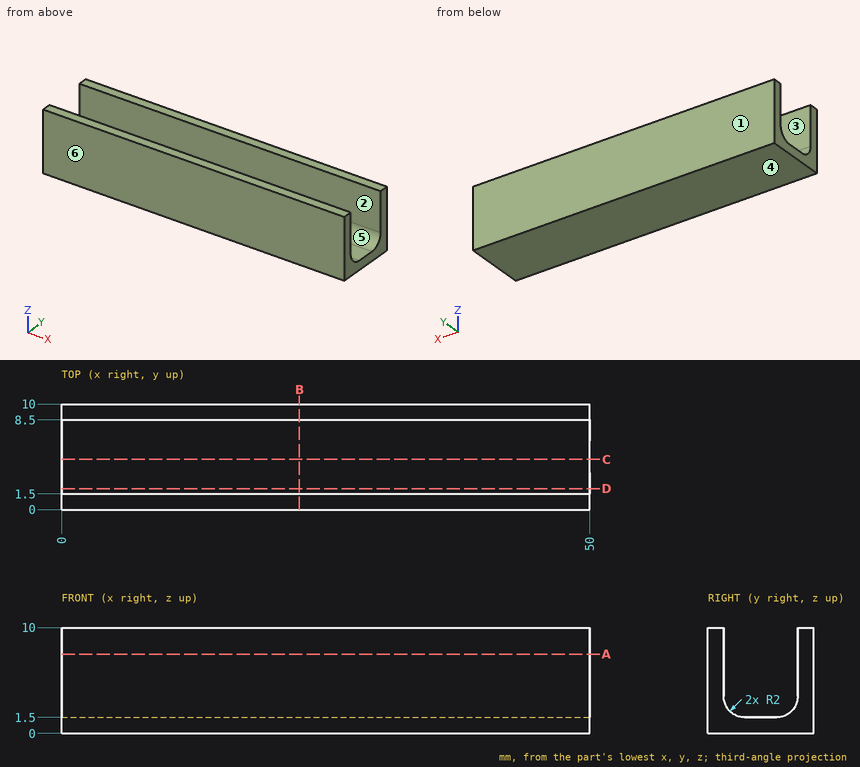
Input: dimensioned drawing with shaded views. Units: mm. Origin: part minimum x, y, z. A direction names the side the tool comes from. Round coordinates to 2 decimals unless told otherwise and drop trailing zeros. Loops run counter-clockwise (first coordinate to the right, second up) from the corner with the lowest first, then second, coordinate; pieces in that order, holes last. Notation, with made-up numbers: (42.25, -13.75) -> (51.25, -13.75) arc R16 ccw to (51.25, 2.25) -> close; hole circle Ø2 at (40, 13.5). An arc over 180 degrees is marked (long way). Answer as a JSON object with one key per item and string values. Group by question number.
Q1. Access query for the marked faces 1 and 2. Directions: +Z, -Z, +X, -X, +Y, -Y. A direction counts if a zero-diameter tool reaches every point of the face in a straight line with its end or side. Return the directions, or none.
Q2. Ray query, line 1 (Y direction, x = 21, z = 6.25); line 2 (Z direction, x = 47, y = 3.75); line 3 (Y direction, x = 17.5, z = 2.5). Return the intervals inside material, ascending. Write a range as from..to.
Q3. Section query A-A (z = 7.5). Output: boundary loops of the cut face in (x, y).
Q4. Section query B-B (x = 22.5). Output: boundary loops of the cut face in (y, z), plus the area to 3 significant figures.
Q5. Mould query, pull axis Y, two halves, no side actions, for the marked faces 3, 4, 5 and 6. Classes: pulls with the +Y half, pulls with the -Y half, needs draft (parallel to the pull), parting line crosses it, or undercut.
Q6. Contact query for a flat-ended pin moving along its axis: P1, Ø2.5, axis at x = 15, y = 5, coming from the +Z side. Output: stop coordinate, or through.
Q7. Section query D-D (y = 2). Output: boundary loops of the cut face in (x, z).
Q8. Section query C-C (y = 4.75). Output: boundary loops of the cut face in (x, z), plus the area to 3 significant figures.
Completed:
{
 "1": {"face 1": "+Z, -Z, +X, -X, +Y", "face 2": "+Z, +X, -X"},
 "2": {"line 1": "0..1.5, 8.5..10", "line 2": "0..1.5", "line 3": "0..1.77, 8.23..10"},
 "3": {"outline": "(0, 0) -> (50, 0) -> (50, 1.5) -> (0, 1.5) -> close; (0, 8.5) -> (50, 8.5) -> (50, 10) -> (0, 10) -> close"},
 "4": {"outline": "(0, 0) -> (10, 0) -> (10, 10) -> (8.5, 10) -> (8.5, 3.5) arc R2 cw to (6.5, 1.5) -> (3.5, 1.5) arc R2 cw to (1.5, 3.5) -> (1.5, 10) -> (0, 10) -> close", "area": "42.2 mm²"},
 "5": {"face 3": "undercut", "face 4": "needs draft", "face 5": "undercut", "face 6": "pulls with the -Y half"},
 "6": {"P1": "z = 1.5"},
 "7": {"outline": "(0, 0) -> (50, 0) -> (50, 2.18) -> (0, 2.18) -> close"},
 "8": {"outline": "(0, 0) -> (50, 0) -> (50, 1.5) -> (0, 1.5) -> close", "area": "75.0 mm²"}
}
